from build123d import *

# Parameters (mm, degrees)
SKETCH4_R           = 2
SKETCH4_R_2         = 1.25
SKETCH4_R_3         = 4.15
SKETCH4_R_4         = 1.75
BOSS_EXTRUDE1_DEPTH = 5.5


with BuildPart() as part:
    # Sketch4 → Boss-Extrude1 (new body)
    with BuildSketch(Plane(origin=(0, 0, 0), x_dir=(1, 0, 0), z_dir=(0, 1, 0))):
        with BuildLine():
            Line((56.335401836, 63.65), (81, 63.65))
            Line((81, 63.65), (81, 57.659411765))
            Line((81, 57.659411765), (80, 57.659411765))
            Line((80, 57.659411765), (79, 58.992745098))
            Line((79, 58.992745098), (77, 58.992745098))
            Line((77, 58.992745098), (77, 55.65))
            Line((77, 55.65), (83, 55.65))
            Line((83, 55.65), (83, 63.65))
            Line((83, 63.65), (85, 63.65))
            Line((85, 63.65), (85, -63.65))
            Line((85, -63.65), (83, -63.65))
            Line((83, -63.65), (83, -55.65))
            Line((83, -55.65), (77, -55.65))
            Line((77, -55.65), (77, -58.992745098))
            Line((77, -58.992745098), (79, -58.992745098))
            Line((79, -58.992745098), (80, -57.659411765))
            Line((80, -57.659411765), (81, -57.659411765))
            Line((81, -57.659411765), (81, -63.65))
            Line((81, -63.65), (56.335401836, -63.65))
            ThreePointArc((56.335401836, -63.65), (0, -85), (-56.335401836, -63.65))
            Line((-56.335401836, -63.65), (-81, -63.65))
            Line((-81, -63.65), (-81, -57.659411765))
            Line((-81, -57.659411765), (-80, -57.659411765))
            Line((-80, -57.659411765), (-79, -58.992745098))
            Line((-79, -58.992745098), (-77, -58.992745098))
            Line((-77, -58.992745098), (-77, -55.65))
            Line((-77, -55.65), (-83, -55.65))
            Line((-83, -55.65), (-83, -63.65))
            Line((-83, -63.65), (-85, -63.65))
            Line((-85, -63.65), (-85, 63.65))
            Line((-85, 63.65), (-83, 63.65))
            Line((-83, 63.65), (-83, 55.65))
            Line((-83, 55.65), (-77, 55.65))
            Line((-77, 55.65), (-77, 58.992745098))
            Line((-77, 58.992745098), (-79, 58.992745098))
            Line((-79, 58.992745098), (-80, 57.659411765))
            Line((-80, 57.659411765), (-81, 57.659411765))
            Line((-81, 57.659411765), (-81, 63.65))
            Line((-81, 63.65), (-56.335401836, 63.65))
            ThreePointArc((-56.335401836, 63.65), (0, 85), (56.335401836, 63.65))
        make_face()
        with Locations(Location((-58, 59.65, 0), (0, 0, 270))):
            Circle(SKETCH4_R, mode=Mode.SUBTRACT)
        with Locations(Location((-66, 59.65, 0), (0, 0, 270))):
            Circle(SKETCH4_R, mode=Mode.SUBTRACT)
        with Locations(Location((66, 59.65, 0), (0, 0, 90))):
            Circle(SKETCH4_R, mode=Mode.SUBTRACT)
        with Locations(Location((58, 59.65, 0), (0, 0, 90))):
            Circle(SKETCH4_R, mode=Mode.SUBTRACT)
        with Locations(Location((66, -59.65, 0), (0, 0, 270))):
            Circle(SKETCH4_R, mode=Mode.SUBTRACT)
        with Locations(Location((58, -59.65, 0), (0, 0, 270))):
            Circle(SKETCH4_R, mode=Mode.SUBTRACT)
        with Locations(Location((-58, -59.65, 0), (0, 0, 90))):
            Circle(SKETCH4_R, mode=Mode.SUBTRACT)
        with Locations(Location((-66, -59.65, 0), (0, 0, 90))):
            Circle(SKETCH4_R, mode=Mode.SUBTRACT)
        with Locations(Location((-16, 16, 0), (0, 0, 270))):
            Circle(SKETCH4_R_2, mode=Mode.SUBTRACT)
        with Locations(Location((16, 16, 0), (0, 0, 270))):
            Circle(SKETCH4_R_2, mode=Mode.SUBTRACT)
        with Locations(Location((16, -16, 0), (0, 0, 270))):
            Circle(SKETCH4_R_2, mode=Mode.SUBTRACT)
        with Locations(Location((-16, -16, 0), (0, 0, 270))):
            Circle(SKETCH4_R_2, mode=Mode.SUBTRACT)
        with Locations(Location((0, 55, 0), (0, 0, 270))):
            Circle(SKETCH4_R_3, mode=Mode.SUBTRACT)
        with Locations(Location((47.631397208, -27.5, 0), (0, 0, 270))):
            Circle(SKETCH4_R_3, mode=Mode.SUBTRACT)
        with Locations(Location((-47.631397208, -27.5, 0), (0, 0, 270))):
            Circle(SKETCH4_R_3, mode=Mode.SUBTRACT)
        with Locations(Location((0, -79.193683245, 0), (0, 0, 270))):
            Circle(SKETCH4_R_4, mode=Mode.SUBTRACT)
        with Locations(Location((-68.58374151, 39.596841623, 0), (0, 0, 270))):
            Circle(SKETCH4_R_4, mode=Mode.SUBTRACT)
        with Locations(Location((68.58374151, 39.596841623, 0), (0, 0, 270))):
            Circle(SKETCH4_R_4, mode=Mode.SUBTRACT)
    extrude(amount=BOSS_EXTRUDE1_DEPTH)


solid = part.part
Model file for the job. Use its own axes, mm. A direction names the side the tool comes from. Coordinates: 2 decimals unless noted, no trailing zeros. Loops run counter-clockwise (first coordinate to the right, second up) from the corner with the lowest first, then second, coordinate; pieces in that order, holes last. Notation, with made-up numbers: (-15.5, -36.5) -> (10.5, -36.5) arc R22 cw to (10.5, -5.5) -> close; hole circle Ø5 at (-21, -17). An arc over 180 degrees is marked (long way). Use one line per item in the form item = value. Start each with the question number.
(1) Cut at B-B on x = 74. Give the cut face in (y, z).
(2) Cut at D-D on z = 70. Give the cut face in (x, y), and give its area (3 significant figures).
(3) Pull direction X, two halves, no side cores. Call faces 1 (the cylindrical face through (-0.862, 2.712, -84.996)), 2 (the flat face through (-68, 3, 63.65)), 3 (the cylindrical face through (-64.648, 2.712, -61.124)): pulls with the +X half, pulls with the -X half, needs draft (parallel to the pull), parting line crosses it, or undercut.
(4) Tool access for faces 4 (the flat face through (-80, 3, -55.65)), 5 (the flat face through (-81, 3, 61)), 6 (the flat face through (81, 3, -61)): list every direction of +Z, -Z, +X, -X, +Y, -Y with a clear straight run to the whole face (end or side of a thin tool).
(5) Probe probe 1 along X at (y, z) = (1.25, 16); probe 2 along X at (y, z) = (2.1, 26.5); probe 3 along Z at (x, y) = (-74.5, 0.9). List the from-to ranges inside material, lowest first. Write a range as from..to.
(6) Cut at C-C on y = 3.1. Give the number of separate pieces and of enclosed holes in the cut face, and give its area (3 significant figures).
(7) Flat gauge pins, fed straight in: pin 1 (6.5 mm diameter, centred on x = 58, z = 59.65, fed in from +Y); pin 2 (3 mm diameter, centred on x = -68.58, z = -39.6, fed in from -Y); pin 3 (1.6 mm diameter, centred on x = -67, y = 2.5, fed in from +Z); pin 4 (2 mm diameter, centred on x = -77.5, y = 2.5, fed in from -Z). Where does each tip first touch, or does it go through?
(8) Cut at A-A on z = 27.5. Give the cut face in (x, y), and give its area (3 significant figures).
Values:
q1.outline = (0, -63.65) -> (5.5, -63.65) -> (5.5, 63.65) -> (0, 63.65) -> close
q2.outline = (-48.22, 0) -> (48.22, 0) -> (48.22, 5.5) -> (-48.22, 5.5) -> close
q2.area = 530 mm2
q3.face_1 = parting line crosses it
q3.face_2 = needs draft
q3.face_3 = undercut
q4.face_4 = +Y, -Y
q4.face_5 = +Z, +Y, -Y
q4.face_6 = -Z, +Y, -Y
q5.probe_1 = -85..-17.25, -14.75..14.75, 17.25..85
q5.probe_2 = -85..-51.66, -43.6..43.6, 51.66..85
q5.probe_3 = -63.65..63.65
q6.separate_pieces = 1
q6.enclosed_holes = 18
q6.area = 24,500 mm2
q7.pin_1 = 5.5
q7.pin_2 = through
q7.pin_3 = 63.65
q7.pin_4 = -63.65
q8.outline = (-85, 0) -> (-51.78, 0) -> (-51.78, 5.5) -> (-85, 5.5) -> close; (-43.48, 0) -> (43.48, 0) -> (43.48, 5.5) -> (-43.48, 5.5) -> close; (51.78, 0) -> (85, 0) -> (85, 5.5) -> (51.78, 5.5) -> close
q8.area = 844 mm2
